from build123d import *

# Parameters (mm, degrees)
SKETCH1_W           = 50.5
SKETCH1_H           = 50.5
BOSS_EXTRUDE1_DEPTH = 42.5
SKETCH1_3_W         = 50.5
SKETCH1_3_H         = 50.5
BOSS_EXTRUDE2_DEPTH = 50
CUT_EXTRUDE1_DEPTH  = 70
CUT_EXTRUDE2_DEPTH  = 70
SKETCH4_R           = 3.1
CUT_EXTRUDE3_DEPTH  = 70
SKETCH5_W           = 35.5
SKETCH5_H           = 50
SKETCH5_W_2         = 7.75
SKETCH5_H_2         = 22.5
CUT_EXTRUDE4_DEPTH  = 55


with BuildPart() as part:
    # Sketch1 → Boss-Extrude1 (new body)
    with BuildSketch(Plane(origin=(0, 0, 0), x_dir=(1, 0, 0), z_dir=(0, 1, 0))):
        Polygon((25.25, 5.5), (30.25, 7.5), (30.25, -7.5), (25.25, -5.5), align=None)
        Rectangle(SKETCH1_W, SKETCH1_H)
    extrude(amount=BOSS_EXTRUDE1_DEPTH)

    # Sketch1_3 → Boss-Extrude2 (add)
    with BuildSketch(Plane(origin=(0, 0, 0), x_dir=(1, 0, 0), z_dir=(0, 1, 0))):
        Rectangle(SKETCH1_3_W, SKETCH1_3_H)
    extrude(amount=-BOSS_EXTRUDE2_DEPTH)

    # Sketch2 → Cut-Extrude1 (cut)
    with BuildSketch(Plane(origin=(0, 0, -25.25), x_dir=(-1, 0, 0), z_dir=(0, 0, -1))):
        Polygon((-5.5, -50), (-7.5, -45), (7.5, -45), (5.5, -50), align=None)
    extrude(amount=-CUT_EXTRUDE1_DEPTH, mode=Mode.SUBTRACT)

    # Sketch3 → Cut-Extrude2 (cut)
    with BuildSketch(Plane(origin=(25.25, 0, 0), x_dir=(0, 0, -1), z_dir=(1, 0, 0))):
        Polygon((17.25, -50), (25.25, -50), (25.25, 0), (17.25, -45), align=None)
    extrude(amount=-CUT_EXTRUDE2_DEPTH, mode=Mode.SUBTRACT)

    # Sketch4 → Cut-Extrude3 (cut)
    with BuildSketch(Plane.XY.offset(25.25)):
        with Locations((0, -25)):
            Circle(SKETCH4_R)
    extrude(amount=-CUT_EXTRUDE3_DEPTH, mode=Mode.SUBTRACT)

    # Sketch5 → Cut-Extrude4 (cut)
    with BuildSketch(Plane.XY.offset(25.25)):
        with Locations((0, 10)):
            Rectangle(SKETCH5_W, SKETCH5_H)
        with Locations((-13.875, -26.25)):
            Rectangle(SKETCH5_W_2, SKETCH5_H_2)
        with Locations((13.875, -26.25)):
            Rectangle(SKETCH5_W_2, SKETCH5_H_2)
    extrude(amount=-CUT_EXTRUDE4_DEPTH, mode=Mode.SUBTRACT)


solid = part.part
Here's how the part is built. I have some questions about the finished solid (model axes, mm). A direction names the side the tool comes from. Give positions to 0.01 mm unless a question says otherwise; leave off trailing zeros. Order: outer loops, then holes, each group sorted by start corner. A loop starts at its lowest first (then second) coordinate and runs counter-clockwise, first axis right, second up. Notation, with made-up numbers: (-1, 42.5) -> (10, 42.5) arc R9 cw to (10, 46.5) -> close; hole circle Ø7 at (34.5, 31). An arc over 180 degrees is marked (long way). Use a Markdown table: item, result. Add a question column.
Item 1: I need wall thicknesses on line 1 (X direction, y = -25, z = -6); line 2 (Y direction, x = 0, z = 7.5); line 3 (X direction, y = -35, z = 17.5). Which ranges of each line are inside material? Lowest first, please.
Item 2: If we mould it in two halves opening along Y, with no side actions, what happens to faces 1 (the face through (15, -50, 4)), 2 (the face through (14, -37.5, 4)), 3 (the face through (-15, -47, -17.25))? For each: pulls with the +Y half, pulls with the -Y half, needs draft (parallel to the pull), parting line crosses it, or undercut.
Item 3: Imagine slicing it at C-C on y = -5.5. Please give me the cut outline in (x, z), plus the area to 3 significant figures.
Item 4: Imagine slicing it at A-A on x = 13. Please give me the cut outline in (y, z).
Item 5: For faces 4 (the face through (27.72, 20.95, -6.49)), 5 (the face through (16, -47, -17.25)), 6 (the face through (-17.75, -1, 0)), which set-ups out of +Z, -Z, +X, -X, +Y, -Y let a thin tool reach every point of the face, with its end or its side?
Item 6: Imagine slicing it at D-D on x = 0. Please give me the cut outline in (y, z), plus the area to 3 significant figures.
Item 7: Imagine slicing it at B-B on y = -25. Please give me the cut outline in (x, z), plus the area to 3 significant figures.
Item 8: Will these pins go through, and if not, where does the flat tip stop? pin 1 (4 mm diameter, centred on x = -20, y = -48.5, fed in from -Z); pin 2 (1.5 mm diameter, centred on x = 29, z = -0.5, fed in from -Y); pin 3 (11 mm diameter, centred on y = -31.5, z = -8.5, fed in from +X); pin 4 (3.5 mm diameter, centred on x = 0, y = -25, fed in from -Z).
Data:
| question | item | result |
|---|---|---|
| 1 | line 1 | x = -25.25 to -17.75, -10 to -3.1, 3.1 to 10, 17.75 to 25.25 |
| 1 | line 2 | y = -45 to -28.1, -21.9 to -15, 35 to 42.5 |
| 1 | line 3 | x = -25.25 to -17.75, -10 to 10, 17.75 to 25.25 |
| 2 | face 1 | pulls with the -Y half |
| 2 | face 2 | undercut |
| 2 | face 3 | needs draft |
| 3 | outline | (-25.25, -24.27) -> (-17.75, -24.27) -> (-17.75, 25.25) -> (-25.25, 25.25) -> close; (17.75, -24.27) -> (25.25, -24.27) -> (25.25, 25.25) -> (17.75, 25.25) -> close |
| 3 | area | 743 mm² |
| 4 | outline | (-50, -17.25) -> (-45, -17.25) -> (-37.5, -18.58) -> (-37.5, 25.25) -> (-50, 25.25) -> close; (35, -25.25) -> (42.5, -25.25) -> (42.5, 25.25) -> (35, 25.25) -> close |
| 5 | face 4 | -Z, +Y, -Y |
| 5 | face 5 | -Z, +X, -X, -Y |
| 5 | face 6 | +Z, -Z |
| 6 | outline | (-45, -17.25) -> (-28.1, -20.25) -> (-28.1, 25.25) -> (-45, 25.25) -> close; (-21.9, -21.36) -> (-15, -22.58) -> (-15, 25.25) -> (-21.9, 25.25) -> close; (35, -25.25) -> (42.5, -25.25) -> (42.5, 25.25) -> (35, 25.25) -> close |
| 6 | area | 1,450 mm² |
| 7 | outline | (-25.25, -20.81) -> (-17.75, -20.81) -> (-17.75, 25.25) -> (-25.25, 25.25) -> close; (-10, -20.81) -> (-3.1, -20.81) -> (-3.1, 25.25) -> (-10, 25.25) -> close; (3.1, -20.81) -> (10, -20.81) -> (10, 25.25) -> (3.1, 25.25) -> close; (17.75, -20.81) -> (25.25, -20.81) -> (25.25, 25.25) -> (17.75, 25.25) -> close |
| 7 | area | 1,330 mm² |
| 8 | pin 1 | stops at z = -17.25 |
| 8 | pin 2 | stops at y = 0 |
| 8 | pin 3 | stops at x = 25.25 |
| 8 | pin 4 | passes through |
